The figure shows three views and two pictorial views of one solid part (mm, origin at its lowest corner). Answer the questions. Round coordinates to 2 decimals unless told otherwise and drop trailing zeros. Write each loop counter-clockwise with the first axis right and the second up, starting at its lowest first coordinate (ties: lowest second). Pieces come first, ordered by that corner, then holes.
Item 1: Find section A-A on z = 29. Give the vertices of the cut face in (x, y), then the cut area to 3 significant figures.
Item 2: For a pull along Z with two mould halves and no side action, classify the marked faces 1 and 2 as +Z half, -Z half, draft (parallel to the pull), parting line (faces both ways), or undercut.
Item 3: Find the intervals of material crossed by probe 1 along Y at (x, z) = (24, 0.7); probe 2 along Z at (x, y) = (14, 2.5); probe 3 along Y at (x, z) = (24, 74.5), in increasing order.
Item 4: Each of these flat-tipped pins is pushed along its axis until it touches: pin 1 (10 mm diameter, centred on x = 17, z = 87.5, fed in from +Y); pin 2 (14.5 mm diameter, centred on x = 17, y = 16, fed in from +Z) (1 decimal); pin 3 (1 mm diameter, centred on x = 25.5, z = 49.5, fed in from -Y); pin 4 (5 mm diameter, centred on y = 32.5, z = 77.5, fed in from -X). Where does it stop, or does it pass through?
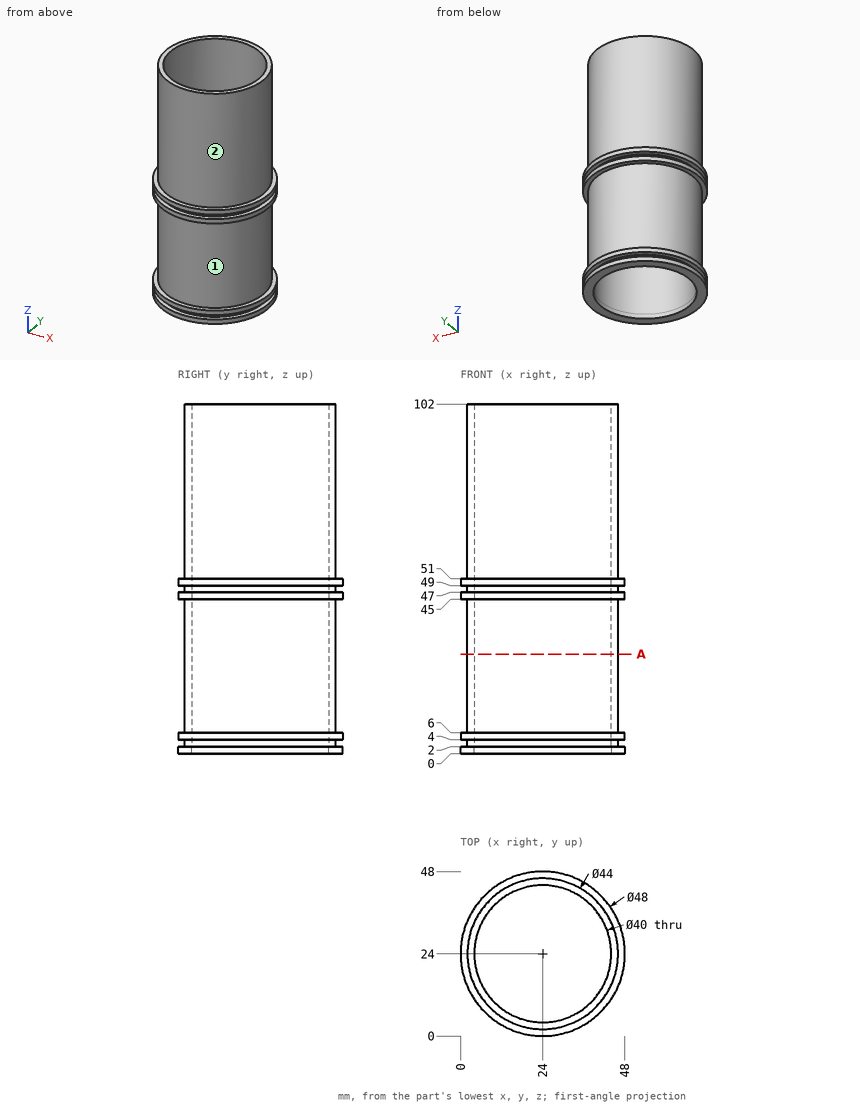
Check values:
1. outline: circle Ø44 at (24, 24); hole circle Ø40 at (24, 24)
1. area: 264 mm2
2. face 1: undercut
2. face 2: draft
3. probe 1: y = 0 to 4, 44 to 48
3. probe 2: z = 0 to 2, 4 to 6, 45 to 47, 49 to 51
3. probe 3: y = 2 to 4, 44 to 46
4. pin 1: stops at y = 45.91
4. pin 2: passes through
4. pin 3: stops at y = 0.02
4. pin 4: stops at x = 2.83
